```python
from build123d import *

# Parameters (mm, degrees)
F0_W      = 140
F0_H      = 70
F1_DEPTH  = 60
F3_DEPTH  = 140
F5_DEPTH  = 70
F6_DEPTH  = 10
F7_W      = 30
F7_H      = 60
F8_DEPTH  = 15
F9_W      = 30
F9_H      = 60
F10_DEPTH = 15


with BuildPart() as f1:
    # F0 (on Top) → F1 (new body)
    with BuildSketch(Plane.XY):
        with Locations((-1.2832614383, 11.7256036028)):
            Rectangle(F0_W, F0_H)
    extrude(amount=F1_DEPTH)

    # F2 (on face) → F3 (cut)
    with BuildSketch(Plane.YZ.offset(68.7167385617)):
        with BuildLine():
            Line((-8.2743963972, 0), (31.7256036028, 0))
            ThreePointArc((31.7256036028, 0), (11.7256036028, 20), (-8.2743963972, 0))
        make_face()
    extrude(amount=-F3_DEPTH, mode=Mode.SUBTRACT)

    # F4 (on face) → F5 (cut)
    with BuildSketch(Plane.XZ.offset(23.2743963972)):
        with BuildLine():
            ThreePointArc((-20, 60), (0, 40), (20, 60))
            Line((20, 60), (-20, 60))
        make_face()
    extrude(amount=-F5_DEPTH, mode=Mode.SUBTRACT)

    # F4 (on face) → F6 (join)
    with BuildSketch(Plane.XZ.offset(23.2743963972)):
        with BuildLine():
            Line((30, 60), (20, 60))
            ThreePointArc((20, 60), (0, 40), (-20, 60))
            Line((-20, 60), (-30, 60))
            ThreePointArc((-30, 60), (0, 30), (30, 60))
        make_face()
    extrude(amount=F6_DEPTH)

    # F7 (on face) → F8 (cut)
    with BuildSketch(Plane.XY.offset(60)):
        with Locations((-56.2832614383, 6.7256036028)):
            Rectangle(F7_W, F7_H)
    extrude(amount=-F8_DEPTH, mode=Mode.SUBTRACT)

    # F9 (on face) → F10 (cut)
    with BuildSketch(Plane.XY.offset(60)):
        with Locations((53.7167385617, 6.7256036028)):
            Rectangle(F9_W, F9_H)
    extrude(amount=-F10_DEPTH, mode=Mode.SUBTRACT)


solid = f1.part
```
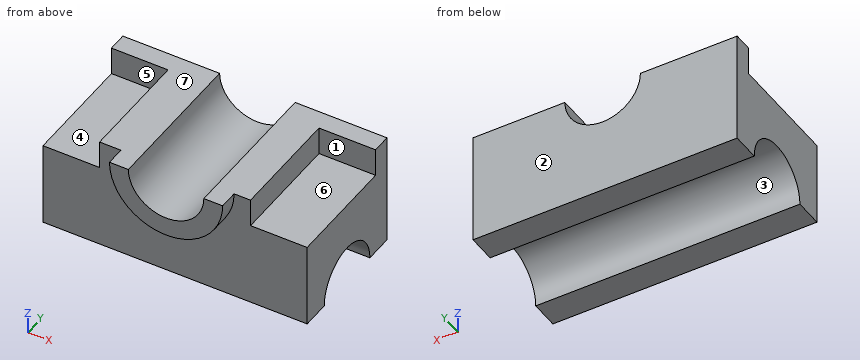
Work out the finished part from the listing and answer in its coordinate system (mm). Face numbers are marked on the shaded views. A direction names the side the tool comes from. Coordinates: 2 decimals unless noted, no trailing zeros. Loops run counter-clockwise (first coordinate to the right, second up) from the corner with the lowest first, then second, coordinate; pieces in that order, holes last. Notation, with made-up numbers: (26, -6.5) - (55, -6.5) arc R4 cw to (55, -1.5) - close; hole circle Ø1 at (-14, -40). An arc over 180 degrees is marked (long way). Use a Markdown table: item, result.
Item 1: For the marked faces 5, 6 and 7, determine the directions among +Z, -Z, +X, -X, +Y, -Y from which every point of the face is accessible in a straight line to the end or side of a thin tool.
Evaluation:
| item | result |
|---|---|
| face 5 | +Z, -X, -Y |
| face 6 | +Z, +X, -Y |
| face 7 | +Z, +X, -X, +Y, -Y |
Item 2: Given pin 1 Ø18 at (x, z) = (31.5, 43.5) entering from -Y; pin 2 Ø7.5 at (y, z) = (1, 54) entering from +X; pin 3 Ø1.5 at (x, z) = (30, 43.5) entering from -Y; pin 4 Ø24 at (x, y) = (-58.5, 11) entering from +Z, each flat-ended and moving along its own axis, determine where each tip first touches the part or whether it passes through.
Evaluation:
| item | result |
|---|---|
| pin 1 | stops at y = -33.27 |
| pin 2 | stops at x = 38.72 |
| pin 3 | stops at y = -23.27 |
| pin 4 | stops at z = 45 |
Item 3: The mould has two halves that part along Y. Classify the marked faces 1, 2, 3 and 4: +Y half, -Y half, draft (parallel to the pull), parting line (faces both ways), or undercut.
Evaluation:
| item | result |
|---|---|
| face 1 | -Y half |
| face 2 | +Y half |
| face 3 | undercut |
| face 4 | draft |
Item 4: Find section C-C, the plane y = -2. Determine the outline of the cut face in (x, z), and give its area (3 significant figures).
Evaluation:
| item | result |
|---|---|
| outline | (-71.28, 14.55) - (68.72, 14.55) - (68.72, 45) - (38.72, 45) - (38.72, 60) - (20, 60) arc R20 cw to (-20, 60) - (-41.28, 60) - (-41.28, 45) - (-71.28, 45) - close |
| area | 4,840 mm2 |
Item 5: Find section B-B, the plane z = 43.5. Determine the outline of the cut face in (x, y).
Evaluation:
| item | result |
|---|---|
| outline | (-71.28, -23.27) - (-25.05, -23.27) - (-25.05, -33.27) - (-11.3, -33.27) - (-11.3, 46.73) - (-71.28, 46.73) - close; (11.3, -33.27) - (25.05, -33.27) - (25.05, -23.27) - (68.72, -23.27) - (68.72, 46.73) - (11.3, 46.73) - close |
Item 6: Find section D-D, the plane x = -60. Determine the outline of the cut face in (y, z).
Evaluation:
| item | result |
|---|---|
| outline | (-23.27, 0) - (-8.27, 0) arc R20 cw to (31.73, 0) - (46.73, 0) - (46.73, 60) - (36.73, 60) - (36.73, 45) - (-23.27, 45) - close |
Item 7: Consider probe 1 along Y at (x, z) = (34.5, 34); probe 2 along Y at (x, z) = (59, 3.5); probe 3 along X at (y, z) = (20, 43.5). Determine where each line is inside the solid, lowest interval first. Write a range as from..to.
Evaluation:
| item | result |
|---|---|
| probe 1 | y = -23.27..46.73 |
| probe 2 | y = -23.27..-7.97, 31.42..46.73 |
| probe 3 | x = -71.28..-11.3, 11.3..68.72 |
Item 8: Find section A-A, the plane x = 0. Determine the outline of the cut face in (y, z), and give its area (3 significant figures).
Evaluation:
| item | result |
|---|---|
| outline | (-33.27, 30) - (-23.27, 30) - (-23.27, 0) - (-8.27, 0) arc R20 cw to (31.73, 0) - (46.73, 0) - (46.73, 40) - (-33.27, 40) - close |
| area | 2,270 mm2 |
